from build123d import *

# Parameters (mm, degrees)
F0_R     = 3.625
F1_DEPTH = 2.75
F3_DEPTH = 1.5
F4_R     = 3.5
F5_DEPTH = 0.5
F7_DEPTH = 3.75
F9_R     = 0.1


# Not quite as in the source:
# - a fillet or chamfer that OpenCascade refuses, or shapes differently, is made with other operations: its cross-section is extruded or revolved along the edge and cut away or added


with BuildPart() as f1:
    # F0 (on Right) → F1 (new body, symmetric)
    with BuildSketch(Plane.YZ):
        Circle(F0_R)
    extrude(amount=F1_DEPTH, both=True)

    # F2 (on face) → F3 (join)
    with BuildSketch(Plane(origin=(-2.75, 0, 0), x_dir=(0, -1, 0), z_dir=(-1, 0, 0))):
        with BuildLine():
            Line((3.5465652398, -0.75), (5.0465652398, -0.75))
            Line((5.0465652398, -0.75), (5.0465652398, 0.75))
            Line((5.0465652398, 0.75), (3.5465652398, 0.75))
            ThreePointArc((3.5465652398, 0.75), (3.625, 0), (3.5465652398, -0.75))
        make_face()
        with BuildLine():
            Line((-3.5465652398, 0.75), (-5.0465652398, 0.75))
            Line((-5.0465652398, 0.75), (-5.0465652398, -0.75))
            Line((-5.0465652398, -0.75), (-3.5465652398, -0.75))
            ThreePointArc((-3.5465652398, -0.75), (-3.625, 0), (-3.5465652398, 0.75))
        make_face()
    extrude(amount=-F3_DEPTH)

    # F4 (on face) → F5 (cut)
    with BuildSketch(Plane.YZ.offset(2.75)):
        Circle(F4_R)
    extrude(amount=-F5_DEPTH, mode=Mode.SUBTRACT)

    # F6 (on face) → F7 (cut)
    with BuildSketch(Plane(origin=(-2.75, 0, 0), x_dir=(0, -1, 0), z_dir=(-1, 0, 0))):
        with BuildLine():
            Line((2.625, -2.5), (-2.625, -2.5))
            ThreePointArc((-2.625, -2.5), (0, -3.625), (2.625, -2.5))
        make_face()
    extrude(amount=-F7_DEPTH, mode=Mode.SUBTRACT)

    # F8: fillet of radius 9 on 1 edges, made by hand

    # F8_s1 → F8_t2 (revolve)
    with BuildSketch(Plane.XY):
        with BuildLine():
            ThreePointArc((2.75, 3.5), (2.3758803254, 2.0419601084), (2.25, 0.5419601084))
            Line((2.25, 0.5419601084), (2.25, 3.5))
            Line((2.25, 3.5), (2.75, 3.5))
        make_face()
    revolve(axis=Axis((2.25, 0, 0), (1, 0, 0)))

    # F9
    f9_edges = [f1.edges().sort_by_distance(p)[0] for p in [
        (2.75, -3.5, 0),
        (2.75, -3.625, 0),
    ]]
    fillet(f9_edges, radius=F9_R)


solid = f1.part
Input: part model. Units: mm. Frame: model coordinates. A direction names the side the tool comes from. Coordinates: 2 decimals unless noted, no trailing zeros. Loops run counter-clockwise (first coordinate to the right, second up) from the corner with the lowest first, then second, coordinate; pieces in that order, holes last.
(1) Set-up query: faces 4 (the face through (-2, -4, 0.75)), 5 (the face through (-1, 0, -2.5)), 6 (the face through (-2, 4, -0.75)). Return all of +Z, -Z, +X, -X, +Y, -Y with unobstructed straight access to the full face (end or side cutting, diameter ignored); none if empty.
(2) First-contact query: pin 1 Ø1.9 at (x, y) = (-1, 1) entering from -Z; pin 2 Ø1.5 at (x, y) = (0.5, 3.5) entering from -Z; pin 3 Ø1 at (x, y) = (1.5, 3) entering from +Z (3 decimals). Flat tips, straight axial feed; report the tip coordinate or a pass-through.
(3) Material intervals for probe 1 along Z at (x, y) = (0, -1); probe 2 along Z at (x, y) = (0.8, 2.5) (3 decimals); probe 3 along X at (y, z) = (2.5, -2), sorted ascending.
(4) Section A-A on x = -1.4. Return the cut outline in (y, z) (3 decimals), then the cut area to 3 significant figures.
(5) Pull-direction query (Z, two-part tool) for faces 1 (the face through (-2.75, 0, 1)), 2 (the face through (2.25, 0, 0)), 3 (the face through (-2, -4, -0.75)); classes: released by +Z, released by -Z, zero draft, split by the parting line, or undercut.
(6) Section C-C on x = -0.4. Return the cut outline in (y, z) (3 decimals), then the cut area to 3 significant figures.
(7) Section B-B on x = 1.45. Return the cut outline in (y, z) (3 decimals), then the cut area to 3 significant figures.
Data:
1. face 4: +Z, +X, -X, -Y
1. face 5: -Z, -X, +Y, -Y
1. face 6: -Z, +X, -X, +Y
2. pin 1: stops at z = -2.5
2. pin 2: stops at z = -2.36
2. pin 3: stops at z = 2.625
3. probe 1: z = -2.5 to 3.48
3. probe 2: z = -2.5 to 2.625
3. probe 3: x = -2.75 to 2.65
4. outline: (-5.047, -0.75) - (-3.547, -0.75) arc R3.625 ccw to (-2.625, -2.5) - (2.625, -2.5) arc R3.625 ccw to (3.547, -0.75) - (5.047, -0.75) - (5.047, 0.75) - (3.547, 0.75) arc R3.625 ccw to (-3.547, 0.75) - (-5.047, 0.75) - close
4. area: 41.5 mm2
5. face 1: zero draft
5. face 2: undercut
5. face 3: released by -Z
6. outline: (-2.625, -2.5) - (2.625, -2.5) arc R3.625 ccw (long way) to start
6. area: 37.2 mm2
7. outline: circle Ø7.25 at (0, 0)
7. area: 41.3 mm2
